The model under review builds one solid part; all positions refer to its coordinate system, in mm. A direction names the side the tool comes from. Give positions to 0.01 mm unless a question says otherwise; leave off trailing zeros. Loops run counter-clockwise (first coordinate to the right, second up) from the corner with the lowest first, then second, coordinate; pieces in that order, holes last. Notation, with made-up numbers: M -7.75,23 L 15.25,23 A21 cw 15.25,48 Z; hole C -22,8 d10. An arc over 180 degrees is marked long. Put each result on its own line as item: value. Start each with the question number.
from build123d import *

# Parameters (mm, degrees)
SKETCH_1_R          = 4
EXTRUDE_1_DEPTH     = 2.2
SKETCH_2_R          = 1.85
EXTRUDE_2_DEPTH     = 10
CHAMFER_1_SIZE      = 0.1
FILLET_1_R          = 0.2
CUT_EXTRUDE_1_DEPTH = 1.5


with BuildPart() as part:
    # Эскиз1 → Бобышка-Вытянуть1 (new body)
    with BuildSketch(Plane(origin=(0, 0, 0), x_dir=(1, 0, 0), z_dir=(0, 1, 0))):
        Circle(SKETCH_1_R)
    extrude(amount=EXTRUDE_1_DEPTH)

    # Эскиз2 → Бобышка-Вытянуть2 (add)
    with BuildSketch(Plane(origin=(0, 2.2, 0), x_dir=(1, 0, 0), z_dir=(0, 1, 0))):
        Circle(SKETCH_2_R)
    extrude(amount=EXTRUDE_2_DEPTH)

    # Фаска1
    chamfer_1_edges = [part.edges().sort_by_distance(p)[0] for p in [
        (-1.85, 12.2, 0),
    ]]
    chamfer(chamfer_1_edges, length=CHAMFER_1_SIZE)

    # Скругление1
    fillet_1_edges = [part.edges().sort_by_distance(p)[0] for p in [
        (-4, 0, 0),
        (-4, 2.2, 0),
    ]]
    fillet(fillet_1_edges, radius=FILLET_1_R)

    # Эскиз3 → Вырез-Вытянуть1 (cut)
    with BuildSketch(Plane.XZ):
        Polygon((-0.5, 0.5), (-0.5, 2), (0.5, 2), (0.5, 0.5), (2, 0.5), (2, -0.5), (0.5, -0.5), (0.5, -2), (-0.5, -2), (-0.5, -0.5), (-2, -0.5), (-2, 0.5), align=None)
    extrude(amount=-CUT_EXTRUDE_1_DEPTH, mode=Mode.SUBTRACT)


solid = part.part
(1) We need section B-B, the plane x = 0. Write out the cut boundary in (y, z), plus the area to 3 significant figures.
(2) We need section C-C, the plane y = 4.75. Write out the cut boundary in (x, z), plus the area to 3 significant figures.
(3) To check wall thickness, follow L1, parallel to Y at x = -1, z = 0; L2, parallel to Y at x = -0.75, z = -2.5; L3, parallel to X at y = 4, z = -0.75. State the ranges of each line that lie inside material, in increasing order. Write a range as [from, to].
(4) Insertion check: pin 1 (0.8 mm diameter, centred on x = 1, y = 1, fed in from -Z); pin 2 (1.2 mm diameter, centred on y = 1, z = 1.5, fed in from -X); pin 3 (1.5 mm diameter, centred on x = 1.5, z = 2, fed in from -Y); pin 4 (0.8 mm diameter, centred on y = 0.5, z = -1.5, fed in from -X). Each pin has a flat end and moves straight along its axis. Give the tip position at first contact, or say it passes through.
(5) We need section A-A, the plane z = 0. Write out the cut boundary in (x, y), plus the area to 3 significant figures.
(6) Draft analysis for pull direction X (two halves, no side actions). For faces 3 (the flat face through (0, 12.2, 0)), 4 (the cylindrical face through (-0.867, 1.087, 3.905)), 5 (the flat face through (-0.5, 1, 1)), state which applies: +X half, -X half, draft (parallel to the pull), parting line (faces both ways), or undercut.
(7) For faces 1 (the cylindrical face through (-0.401, 7.081, 1.806)), 2 (the flat face through (-0.5, 1, -1)), list the 3-axis set-ups (+Z, -Z, +X, -X, +Y, -Y) from which the entire face can be reached by the end or side of a thin tool; tool diameter is ignored.
Check sheet entries:
1. outline: M 0,-3.8 A0.2 ccw 0.2,-4 L 2,-4 A0.2 ccw 2.2,-3.8 L 2.2,-1.85 L 12.1,-1.85 L 12.2,-1.75 L 12.2,1.75 L 12.1,1.85 L 2.2,1.85 L 2.2,3.8 A0.2 ccw 2,4 L 0.2,4 A0.2 ccw 0,3.8 L 0,2 L 1.5,2 L 1.5,-2 L 0,-2 Z
1. area: 48.6 mm²
2. outline: C 0,0 d3.7
2. area: 10.8 mm²
3. L1: y = [1.5, 12.2]
3. L2: y = [0, 2.2]
3. L3: x = [-1.69, 1.69]
4. pin 1: stops at z = -3.95
4. pin 2: stops at x = -3.9
4. pin 3: stops at y = 0
4. pin 4: stops at x = -3.85
5. outline: M -4,0.2 A0.2 ccw -3.8,0 L -2,0 L -2,1.5 L 2,1.5 L 2,0 L 3.8,0 A0.2 ccw 4,0.2 L 4,2 A0.2 ccw 3.8,2.2 L 1.85,2.2 L 1.85,12.1 L 1.75,12.2 L -1.75,12.2 L -1.85,12.1 L -1.85,2.2 L -3.8,2.2 A0.2 ccw -4,2 Z
5. area: 48.6 mm²
6. face 3: draft
6. face 4: parting line
6. face 5: undercut
7. face 1: +Y
7. face 2: -Y
